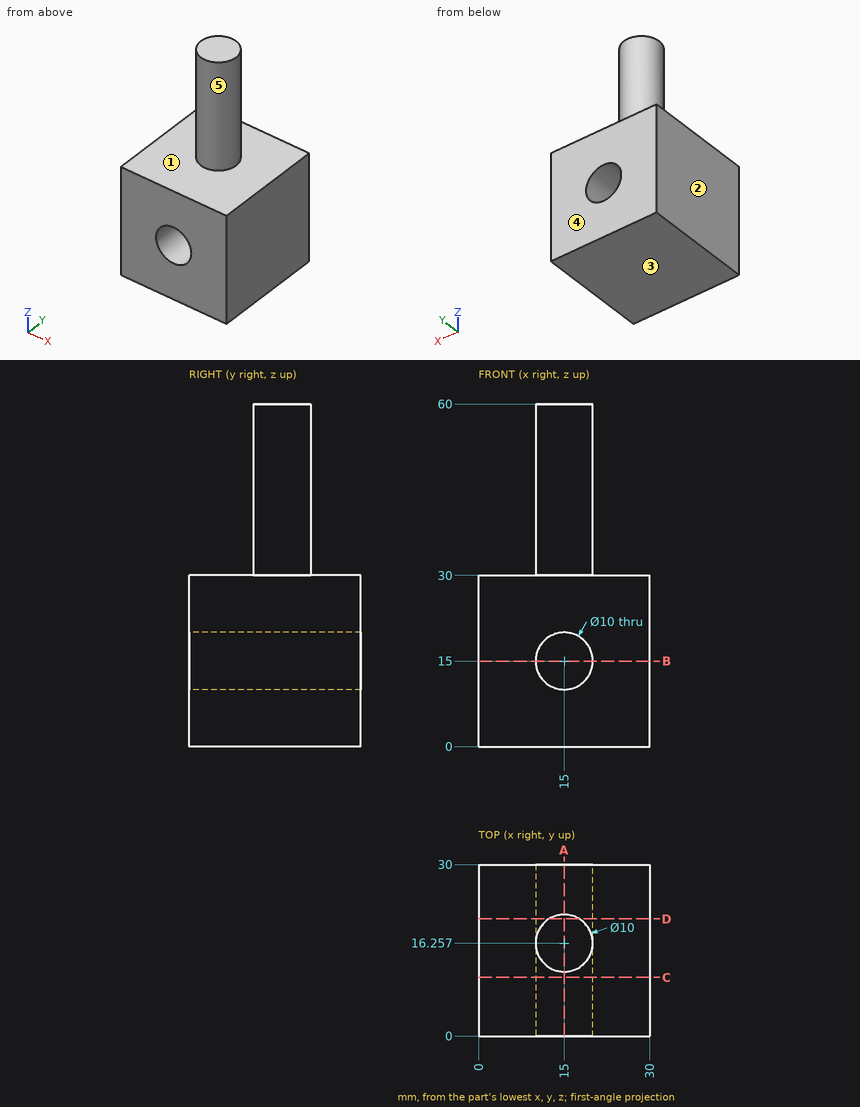
Verification items for this drawing (mm, ordinates from the low corner). A direction names the side the tool comes from. Give positions to 0.01 mm unless a question says otherwise; leave off trailing zeros. Loops run counter-clockwise (first coordinate to the right, second up) from the corner with the lowest first, then second, coordinate; pieces in that order, holes last. Notation, with made-up numbers: M 46.5,-28.75 L 86.5,-28.75 A21 ccw 86.5,-13.75 Z; hole C 32,36.5 d5. An arc over 180 degrees is marked long. Answer as a JSON object with one key per item and string values. Group by question number.
Item 1: Sectioned sample at A-A on x = 15. Record the boundary of the cut face in (y, z), plus the area to 3 significant figures.
Item 2: Mould release check, pull along Y, two halves, no side actions. Record for the marked faces 3, 4 and 5: pulls with the +Y half, pulls with the -Y half, needs draft (parallel to the pull), parting line crosses it, or undercut.
Item 3: Sectioned sample at C-C on y = 10.25. Record the boundary of the cut face in (x, z).
Item 4: Material ranges on L1, parallel to Z at x = 15, y = 18.75; L2, parallel to Z at x = 15, y = 6.25; L3, parallel to Z at x = 6.75, y = 25.5, recorded low to high.
Item 5: Access from +Z, -Z, +X, -X, +Y, -Y to the whole of each face (thin tool, end or side, straight path). Record for the marked faces 1 and 2.
Item 6: Gauge pin test, flat ends, axial feed: pin 1 (5 mm diameter, centred on x = 15.5, z = 45, fed in from +Y); pin 2 (3 mm diameter, centred on y = 20, z = 32.5, fed in from -X); pin 3 (1 mm diameter, centred on y = 20.5, z = 34.5, fed in from -X) (1 decimal). Record the tip position at first contact, or that the pin passes through.
Item 7: Sectioned sample at D-D on y = 20.5. Record the boundary of the cut face in (x, z) (1 decimal), plus the area to 3 significant figures.
Item 8: Sectioned sample at B-B on z = 15. Record the boundary of the cut face in (x, y).
Findings below:
{
 "1": {"outline": "M 0,0 L 30,0 L 30,10 L 0,10 Z; M 0,20 L 30,20 L 30,30 L 21.26,30 L 21.26,60 L 11.26,60 L 11.26,30 L 0,30 Z", "area": "900 mm2"},
 "2": {"face 3": "needs draft", "face 4": "pulls with the +Y half", "face 5": "parting line crosses it"},
 "3": {"outline": "M 0,0 L 30,0 L 30,30 L 0,30 Z; hole C 15,15 d10"},
 "4": {"L1": "0 to 10, 20 to 60", "L2": "0 to 10, 20 to 30", "L3": "0 to 30"},
 "5": {"face 1": "+Z", "face 2": "+Z, -Z, -X, +Y, -Y"},
 "6": {"pin 1": "y = 21.26", "pin 2": "x = 10.53", "pin 3": "x = 11.7"},
 "7": {"outline": "M 0,0 L 30,0 L 30,30 L 17.6,30 L 17.6,60 L 12.4,60 L 12.4,30 L 0,30 Z; hole C 15,15 d10", "area": "980 mm2"},
 "8": {"outline": "M 0,0 L 10,0 L 10,30 L 0,30 Z; M 20,0 L 30,0 L 30,30 L 20,30 Z"}
}
